Part model, mm, in its own coordinate system. Coordinates: 2 decimals unless noted, no trailing zeros. Order: outer loops, then holes, each group sorted by start corner. A loop starts at its lowest first (then second) coordinate and runs counter-clockwise, first axis right, second up. Notation, with made-up numbers: M 45,58.5 L 76,58.5 A34 cw 76,89.5 Z; hole C 22,-14.5 d4. An arc over 180 degrees is marked long. Write item = value, one per line. Start each with the question number.
from build123d import *

# Parameters (mm, degrees)
SKETCH1_R           = 22
SKETCH1_R_2         = 0.6
SKETCH1_R_3         = 1.125
BOSS_EXTRUDE1_DEPTH = 7
FILLET1_R           = 1


with BuildPart() as part:
    # Sketch1 → Boss-Extrude1 (new body)
    with BuildSketch(Plane(origin=(0, 0, 0), x_dir=(1, 0, 0), z_dir=(0, 1, 0))):
        with Locations(Location((0, 0, 0), (0, 0, 270))):
            Circle(SKETCH1_R)
        with Locations(Location((-4, 14, 0), (0, 0, 270))):
            Circle(SKETCH1_R_2, mode=Mode.SUBTRACT)
        with Locations(Location((-4, -14, 0), (0, 0, 270))):
            Circle(SKETCH1_R_2, mode=Mode.SUBTRACT)
        with Locations(Location((15, 0, 0), (0, 0, 270))):
            Circle(SKETCH1_R_2, mode=Mode.SUBTRACT)
        with Locations(Location((-9, 0, 0), (0, 0, 270))):
            Circle(SKETCH1_R_3, mode=Mode.SUBTRACT)
        with Locations(Location((4.5, 7.8, 0), (0, 0, 270))):
            Circle(SKETCH1_R_3, mode=Mode.SUBTRACT)
        with Locations(Location((4.5, -7.8, 0), (0, 0, 270))):
            Circle(SKETCH1_R_3, mode=Mode.SUBTRACT)
    extrude(amount=BOSS_EXTRUDE1_DEPTH)

    # Fillet1
    fillet1_edges = [part.edges().sort_by_distance(p)[0] for p in [
        (0, 0, -22),
    ]]
    fillet(fillet1_edges, radius=FILLET1_R)


solid = part.part
Item 1: Pull direction X, two halves, no side cores. Call faces 1 (the cylindrical face through (-21.477, 3.958, -4.769)), 2 (the flat face through (0, 7, 0)), 3 (the cylindrical face through (-3.82, 3.451, 14.572)): pulls with the +X half, pulls with the -X half, needs draft (parallel to the pull), parting line crosses it, or undercut.
Item 2: Flat gauge pins, fed straight in: pin 1 (1.5 mm diameter, centred on y = 6.5, z = 14.5, fed in from +X); pin 2 (1.1 mm diameter, centred on x = -4, z = -14, fed in from -Y); pin 3 (10 mm diameter, centred on x = 14.5, z = 0, fed in from -Y); pin 4 (4 mm diameter, centred on x = 13.5, y = 5.5, fed in from -Z) (3 decimals). Where does each tip first touch, or does it go through?
Item 3: Wall check: line 1 along X through (y, z) = (2.5, 0) (3 decimals); line 2 along Z through (x, y) = (3.5, 1.75); line 3 along X through (y, z) = (0.5, 8.5). Give the ranges that are in metal, low to high. Write a range as [from, to].
Item 4: Cut at A-A, the plane y = 6.25. Write the cut outline in (x, z) (3 decimals).
Item 5: Cut at B-B, the plane x = 4.5. Count the separate pieces of the cut face and the enclosed holes in it, and give its area (3 significant figures).
Filled sheet:
q1.face_1 = parting line crosses it
q1.face_2 = needs draft
q1.face_3 = undercut
q2.pin_1 = 17.17
q2.pin_2 = through
q2.pin_3 = 0
q2.pin_4 = -18.755
q3.line_1 = [-22, -10.125], [-7.875, 14.4], [15.6, 22]
q3.line_2 = [-21.72, -8.32], [-7.28, 7.28], [8.32, 21.72]
q3.line_3 = [-20.15, 3.62], [5.38, 20.15]
q4.outline = C 0,0 d44; hole C -9,0 d2.25; hole C -4,-14 d1.2; hole C -4,14 d1.2; hole C 4.5,-7.8 d2.25; hole C 4.5,7.8 d2.25; hole C 15,0 d1.2
q5.separate_pieces = 3
q5.enclosed_holes = 0
q5.area = 270 mm2
